Autodesk Inventor part; units mm, degrees
ref_plane "YZ Plane" through (0, 0, 0) normal (1, 0, 0) x (0, 1, 0)
ref_plane "XZ Plane" through (0, 0, 0) normal (0, 1, 0) x (-1, 0, 0)
ref_plane "XY Plane" through (0, 0, 0) normal (0, 0, 1) x (1, 0, 0)
sketch "Sketch1" plane through (0, 0, 0) normal (1, 0, 0) x (0, 1, 0)
  line L0 (25, 748.8121) -> (0, 748.8121)
  line L1 (0, 748.8121) -> (0, -748.8121)
  line L2 (0, -748.8121) -> (25, -748.8121)
  arc A0 (25, -748.8121) -> (25, 748.8121) centre (-5575.159, 0) ccw
  line L3 (0, 748.8121) -> (25.2835, 746.689)
  line L4 (0, -748.8121) -> (25.2835, -746.689)
  line L5 (0, 97) -> (74.0083, 97)
  point P0 (0, 0)
  point P1 (0, 0)
  dimension "d2" = 25
  dimension "d3" = 5650
  dimension "d7" = 85.2
  dimension "d8" = 85.2
  dimension "d33" = 97
  dimension "d34" = 651.812
extrude "Plate1" add sketch "Sketch1" against normal blind 3 contours L3 A0 L5 L1
fillet "Corner Round3" radius 10 1 edges at (-1.5, 25.2835, 746.689)
sketch "Sketch4" plane through (0, 0, 0) normal (1, 0, 0) x (0, 0, -1)
  circle A0 centre (-735.8121, 10) radius 3.5
  line L0 (-748.8121, 0) -> (-97, 0)
  point P0 (0, 0)
  dimension "d23" = 7
  dimension "d25" = 10
  dimension "d32" = 13
extrude "Extrusion1" cut sketch "Sketch4" against normal through all
pattern_linear "Rectangular Pattern2" count 6 spacing 72.5 along (0, 0, -1) of "Extrusion1"
equation "\"d4\" = Thickness"
equation "\"BendReliefWidth\" = Thickness"
equation "\"BendReliefDepth\" = 0.5 * Thickness"
equation "\"CornerReliefSize\" = 4 * Thickness"
equation "\"MinimumRemnant\" = 2 * Thickness"
equation "\"TransitionRadius\" = BendRadius"
equation "\"JacobiRadiusSize\" = BendRadius"
equation "\"GapSize\" = Thickness"
properties part number "MSC 812 TOP SUPPORT GILLS" material "Stainless Steel"
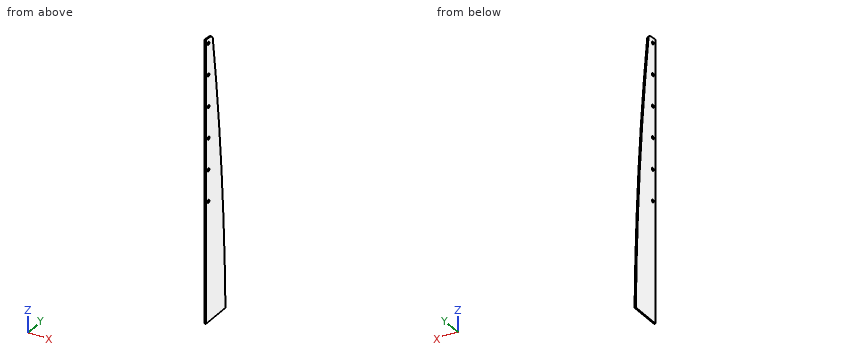
Verification items for the finished model (mm, model axes). Give positions to 0.01 mm unless a question says otherwise; leave off trailing zeros. Write each loop counter-clockwise with the first axis right and the second up, starting at its lowest first coordinate (ties: lowest second). Pieces come first, ordered by that corner, then holes. Notation, with made-up numbers: (27.5, 60.25) -> (46.5, 60.25) arc R18 ccw to (46.5, 70.25) -> close; hole circle Ø4 at (76, 40.25). An arc over 180 degrees is marked (long way). Use CSV: the item, a comma, the result in double quotes.
(1) Go/stop test with flat-tipped pins: pin 1 (4 mm diameter, centred on y = 10, z = 663.31, fed in from -X); pin 2 (1 mm diameter, centred on x = -2, y = 25.5, fed in from +Z). Record where each tip stops, or that it passes through.
Derived:
pin 1,"passes through"
pin 2,"stops at z = 742.55"
(2) Sectioned sample at A-A (x = -1.35). Record the cut outline in (y, z).
Derived:
outline,"(0, 97) -> (74.01, 97) arc R5650 ccw to (26.34, 738.7) arc R10 ccw to (17.26, 747.36) -> (0, 748.81) -> close; hole circle Ø7 at (10, 373.31); hole circle Ø7 at (10, 445.81); hole circle Ø7 at (10, 518.31); hole circle Ø7 at (10, 590.81); hole circle Ø7 at (10, 663.31); hole circle Ø7 at (10, 735.81)"
(3) Sectioned sample at C-C (z = 296.5). Record the cut outline in (x, y), plus the area to 3 significant figures.
Derived:
outline,"(-3, 0) -> (0, 0) -> (0, 67.06) -> (-3, 67.06) -> close"
area,"201 mm^2"
(4) Material ranges on L1, parallel to Y at x = -2.75, z = 271.5; L2, parallel to Y at x = -2.6, z = 478, recorded low to high.
Derived:
L1,"y = 0 to 68.31"
L2,"y = 0 to 54.58"
